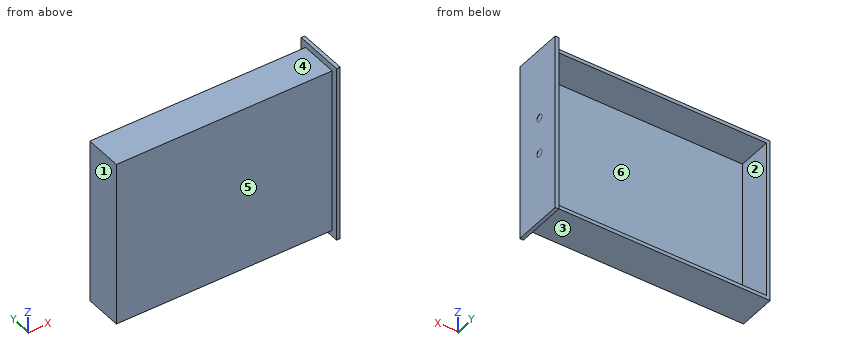
from build123d import *

# Parameters (mm, degrees)
SKETCH1_W           = 487.8
SKETCH1_H           = 137.7
SKETCH1_W_2         = 453.8
SKETCH1_H_2         = 103.7
BOSS_EXTRUDE2_DEPTH = 10
BOSS_EXTRUDE3_DEPTH = 600
SKETCH5_W           = 433.8
SKETCH5_H           = 93.7
BOSS_EXTRUDE4_DEPTH = 10
SKETCH6_W           = 453.8
SKETCH6_H           = 103.7
BOSS_EXTRUDE5_DEPTH = 10
SKETCH7_R           = 25
CUT_EXTRUDE2_DEPTH  = 5
SKETCH8_W           = 116.599055382
SKETCH8_H           = 75.38732029
BOSS_EXTRUDE6_DEPTH = 9
SKETCH9_R           = 10
CUT_EXTRUDE4_DEPTH  = 0.5


with BuildPart() as part:
    # Sketch1 → Boss-Extrude2 (new body)
    with BuildSketch(Plane(origin=(0, 0, 0), x_dir=(0, 0, -1), z_dir=(1, 0, 0))):
        with Locations((124.007003891, -7.666536965)):
            Rectangle(SKETCH1_W, SKETCH1_H)
        with Locations((124.007003891, -7.666536965)):
            Rectangle(SKETCH1_W_2, SKETCH1_H_2, mode=Mode.SUBTRACT)
    extrude(amount=-BOSS_EXTRUDE2_DEPTH)

    # Sketch4 → Boss-Extrude3 (add)
    with BuildSketch(Plane(origin=(0, 0, 0), x_dir=(0, 0, -1), z_dir=(1, 0, 0))):
        Polygon((-92.892996109, -49.516536965), (-92.892996109, 34.183463035), (-92.892996109, 44.183463035), (-102.892996109, 44.183463035), (-102.892996109, -59.516536965), (350.907003891, -59.516536965), (350.907003891, 44.183463035), (340.907003891, 44.183463035), (340.907003891, 34.183463035), (340.907003891, -49.516536965), align=None)
    extrude(amount=-BOSS_EXTRUDE3_DEPTH)

    # Sketch5 → Boss-Extrude4 (add)
    with BuildSketch(Plane(origin=(0, 0, 0), x_dir=(0, 0, -1), z_dir=(1, 0, 0))):
        with Locations((124.007003891, -2.666536965)):
            Rectangle(SKETCH5_W, SKETCH5_H)
    extrude(amount=-BOSS_EXTRUDE4_DEPTH)

    # Sketch6 → Boss-Extrude5 (add)
    with BuildSketch(Plane.ZY.offset(600)):
        with Locations((-124.007003891, -7.666536965)):
            Rectangle(SKETCH6_W, SKETCH6_H)
    extrude(amount=-BOSS_EXTRUDE5_DEPTH)

    # Sketch7 → Cut-Extrude2 (cut)
    with BuildSketch(Plane(origin=(0, 0, 0), x_dir=(0, 0, -1), z_dir=(1, 0, 0))):
        with Locations((124.007003891, -11.609012226)):
            Circle(SKETCH7_R)
    extrude(amount=-CUT_EXTRUDE2_DEPTH, mode=Mode.SUBTRACT)

    # Sketch8 → Boss-Extrude6 (add)
    with BuildSketch(Plane(origin=(0, 0, 0), x_dir=(0, 0, -1), z_dir=(1, 0, 0))):
        with Locations((135.566393002, -11.938485115)):
            Rectangle(SKETCH8_W, SKETCH8_H)
    extrude(amount=-BOSS_EXTRUDE6_DEPTH)

    # Sketch9 → Cut-Extrude4 (cut)
    with BuildSketch(Plane(origin=(0, 0, 0), x_dir=(0, 0, -1), z_dir=(1, 0, 0))):
        with Locations((74.007003891, 0)):
            Circle(SKETCH9_R)
        with Locations((174.007003891, 0)):
            Circle(SKETCH9_R)
    extrude(amount=-CUT_EXTRUDE4_DEPTH, mode=Mode.SUBTRACT)


solid = part.part
Can you work these out from the model? Positions are in its coordinate system, mm. Face numbers are marked on the shaded views. A direction names the side the tool comes from. Give positions to 0.01 mm unless a question says otherwise; leave off trailing zeros. Order: outer loops, then holes, each group sorted by start corner. A loop starts at its lowest first (then second) coordinate and runs counter-clockwise, first axis right, second up. Notation, with made-up numbers: M 57,-38 L 77,-38 A9 cw 77,-29 Z; hole C 25.25,88.5 d1. An arc over 180 degrees is marked long. Use one line per item in the form item = value.
Item 1: Thinking about a two-plate mould opening in Z: for the marked faces 4, 5 and 6, which applies, pulls with the +Z half, pulls with the -Z half, needs draft (parallel to the pull), parting line crosses it, or undercut?
Values follow:
face_4 = pulls with the +Z half
face_5 = needs draft
face_6 = undercut
Item 2: Will these pins go through, and if not, where does the flat tip stop? pin 1 Ø16 at (y, z) = (1.5, -175) entering from +X; pin 2 Ø2 at (x, y) = (-505, -34.5) entering from +Z; pin 3 Ø2 at (x, z) = (-173.5, -150.5) entering from +Y.
Values follow:
pin_1 = -0.5
pin_2 = 102.89
pin_3 = -49.52
Item 3: If I drill on line 1 along Z through (x, y) = (-331, 39.5); line 2 along X through (y, z) = (-8, -40); line 3 along Y through (x, z) = (-231.5, -92), over which ranges is the centre line in solid material (lowest first)? Write a range as [from, to].
Values follow:
line_1 = [-350.91, -340.91], [92.89, 102.89]
line_2 = [-600, -590], [-10, 0]
line_3 = [-59.52, -49.52]
Item 4: If we section it at C-C, the plane x = -324.5: Write out the boundary of the cut face in (y, z), and give its area (3 significant figures).
Values follow:
outline = M -59.52,-350.91 L 44.18,-350.91 L 44.18,-340.91 L -49.52,-340.91 L -49.52,92.89 L 44.18,92.89 L 44.18,102.89 L -59.52,102.89 Z
area = 6,410 mm^2
Item 5: If we section it at B-B, the plane z = -305: Write out the boundary of the cut face in (x, y).
Values follow:
outline = M -600,-59.52 L -10,-59.52 L -10,-76.52 L 0,-76.52 L 0,61.18 L -10,61.18 L -10,-49.52 L -590,-49.52 L -590,44.18 L -600,44.18 Z
Item 6: For the marked faces 1, 2 and 3, which set-ups out of +Z, -Z, +X, -X, +Y, -Y let a thin tool reach every point of the face, with its end or its side?
Values follow:
face_1 = +Z, -Z, -X, +Y, -Y
face_2 = +Y
face_3 = -Z, -X, +Y, -Y
Item 7: If we section it at A-A, the plane y = 24.5: Write out the boundary of the cut face in (x, z), and give its area (3 significant figures).
Values follow:
outline = M -600,-350.91 L -10,-350.91 L -10,-367.91 L 0,-367.91 L 0,119.89 L -10,119.89 L -10,102.89 L -600,102.89 Z; hole M -590,-340.91 L -10,-340.91 L -10,92.89 L -590,92.89 Z
area = 21,000 mm^2
Item 8: If we section it at D-D, the plane y = 53.5: Write out the boundary of the cut face in (x, z), and give its area (3 significant figures).
Values follow:
outline = M -10,-367.91 L 0,-367.91 L 0,119.89 L -10,119.89 Z
area = 4,880 mm^2
